```python
from build123d import *

# Parameters (mm, degrees)
SKETCH1_R           = 4.6736
BOSS_EXTRUDE1_DEPTH = 3.302
SKETCH2_R           = 6.096
BOSS_EXTRUDE2_DEPTH = 2.032
CHAMFER1_SIZE       = 0.762
CHAMFER2_SIZE       = 0.508


with BuildPart() as part:
    # Sketch1 → Boss-Extrude1 (new body)
    with BuildSketch(Plane(origin=(0, 0, 0), x_dir=(1, 0, 0), z_dir=(0, 1, 0))):
        with Locations(Location((0, 0, 0), (0, 0, 90))):
            Circle(SKETCH1_R)
    extrude(amount=BOSS_EXTRUDE1_DEPTH)

    # Sketch2 → Boss-Extrude2 (add)
    with BuildSketch(Plane(origin=(0, 3.302, 0), x_dir=(1, 0, 0), z_dir=(0, 1, 0))):
        with Locations(Location((0, 0, 0), (0, 0, 270))):
            Circle(SKETCH2_R)
    extrude(amount=BOSS_EXTRUDE2_DEPTH)

    # Chamfer1
    chamfer1_edges = [part.edges().sort_by_distance(p)[0] for p in [
        (0, 5.334, -6.096),
    ]]
    chamfer(chamfer1_edges, length=CHAMFER1_SIZE)

    # Chamfer2
    chamfer2_edges = [part.edges().sort_by_distance(p)[0] for p in [
        (0, 0, 4.6736),
    ]]
    chamfer(chamfer2_edges, length=CHAMFER2_SIZE)


solid = part.part
```
Source: CAD feature listing. Evaluate the final solid. Frame: model axes, mm. A direction names the side the tool comes from. Coordinates: 2 decimals unless noted, no trailing zeros. Loops run counter-clockwise (first coordinate to the right, second up) from the corner with the lowest first, then second, coordinate; pieces in that order, holes last. Notation, with made-up numbers: (36, -34.5) -> (81, -34.5) arc R21 ccw to (81, -22.5) -> close; hole circle Ø7 at (66, 7.25). An arc over 180 degrees is marked (long way). One line per item, written item: value. Start each with the question number.
Q1. Line query: line 1 along Y through (x, z) = (-3.75, 3.75); line 2 along X through (y, z) = (2.85, 3.75); line 3 along Z through (x, y) = (-0.75, 3.15). Output: solid intervals per line, ascending.
Q2. Section query A-A, the plane x = 0. Return the cut outline in (y, z).
Q3. Contact query for flat-ended pins moving along their axis: P1, Ø2, axis at x = -4.5, y = 1, coming from the +Z side; P2, Ø3, axis at x = -1, y = 3.5, coming from the +Z side. Output: stop coordinate, or through.
Q4. Section query D-D, the plane y = 2.4. Return the cut outline in (x, z), and give its area (3 significant figures).
Q5. Set-up query: faces 1 (the face through (0, 5.334, 0)), 2 (the face through (4.146, 1.885, -2.157)). Return all of +Z, -Z, +X, -X, +Y, -Y with unobstructed straight access to the full face (end or side cutting, diameter ignored); none if empty.
Q6. Section query B-B, the plane z = 0. Return the cut outline in (x, y), and give its area (3 significant figures).
Q7. Section query C-C, the plane y = 3.9. Return the cut outline in (x, z).
Results:
1. line 1: 3.3 to 5.33
1. line 2: -2.79 to 2.79
1. line 3: -4.61 to 4.61
2. outline: (0, -4.17) -> (0.51, -4.67) -> (3.3, -4.67) -> (3.3, -6.1) -> (4.57, -6.1) -> (5.33, -5.33) -> (5.33, 5.33) -> (4.57, 6.1) -> (3.3, 6.1) -> (3.3, 4.67) -> (0.51, 4.67) -> (0, 4.17) -> close
3. P1: z = 3.1
3. P2: z = 6.1
4. outline: circle Ø9.35 at (0, 0)
4. area: 68.6 mm^2
5. face 1: +Z, -Z, +X, -X, +Y
5. face 2: -Y
6. outline: (-6.1, 3.3) -> (-4.67, 3.3) -> (-4.67, 0.51) -> (-4.17, 0) -> (4.17, 0) -> (4.67, 0.51) -> (4.67, 3.3) -> (6.1, 3.3) -> (6.1, 4.57) -> (5.33, 5.33) -> (-5.33, 5.33) -> (-6.1, 4.57) -> close
6. area: 54.8 mm^2
7. outline: circle Ø12.19 at (0, 0)
